Check sheet for the modelled part. Datum: model origin and axes. Units: mm. A direction names the side the tool comes from. Give positions to 0.01 mm unless a question says otherwise; leave off trailing zeros. Write each loop counter-clockwise with the first axis right and the second up, starting at its lowest first coordinate (ties: lowest second). Pieces come first, ordered by that corner, then holes. Notation, with made-up numbers: (-30.75, 60) -> (15.25, 60) arc R26 cw to (15.25, 79) -> close; hole circle Ø11 at (-10.5, 60.5). An arc over 180 degrees is marked (long way). Answer as a JSON object with one key per item and string values.
from build123d import *

# Parameters (mm, degrees)
SKETCH1_W            = 127
SKETCH1_H            = 101.6
BOSS_EXTRUDE1_DEPTH  = 76.2
SKETCH2_R            = 6.35
BOSS_EXTRUDE3_DEPTH  = 50.8
LPATTERN2_COUNT      = 3
LPATTERN2_PITCH      = 15.24
LPATTERN2_COUNT_DIR2 = 3
LPATTERN2_PITCH_DIR2 = 15.24


with BuildPart() as part:
    # Sketch1 → Boss-Extrude1 (new body)
    with BuildSketch(Plane.XY):
        with Locations((63.5, -50.8)):
            Rectangle(SKETCH1_W, SKETCH1_H)
    extrude(amount=BOSS_EXTRUDE1_DEPTH)

    # Sketch2 → Boss-Extrude3 (add)
    with BuildSketch(Plane(origin=(0, 0, 0), x_dir=(1, 0, 0), z_dir=(0, 1, 0))):
        with Locations(Location((68.819241674, -37.547351514, 0), (0, 0, 90))):
            Circle(SKETCH2_R)
    boss_extrude3 = extrude(amount=BOSS_EXTRUDE3_DEPTH)

    # LPattern2: Boss-Extrude3 3 × 3, 1 skipped
    with Locations(*[(-i * LPATTERN2_PITCH, 0, j * LPATTERN2_PITCH_DIR2) for i in range(LPATTERN2_COUNT) for j in range(LPATTERN2_COUNT_DIR2) if (i, j) not in ((0, 0), (1, 1))]):
        add(boss_extrude3)


solid = part.part
1. Access from +Z, -Z, +X, -X, +Y, -Y to the whole of each face (thin tool, end or side, straight path). Record for faces 4 (the face through (53, 50.8, 68)), 5 (the face through (75, 25, 39)).
Determined:
{"face 4": "+Z, -Z, +X, -X, +Y", "face 5": "+Y"}
2. Sectioned sample at D-D, the plane z = 48.5. Enter the section's corners in (x, y).
Determined:
{"outline": "(0, -101.6) -> (127, -101.6) -> (127, 0) -> (73.5, 0) -> (73.5, 50.8) -> (64.14, 50.8) -> (64.14, 0) -> (43.02, 0) -> (43.02, 50.8) -> (33.66, 50.8) -> (33.66, 0) -> (0, 0) -> close"}
3. Scan lines: L1, parallel to X at y = 6, z = 40.5; L2, parallel to Y at x = 22, z = 18. Record each from-to range of solid material in increasing order. Write a range as [from, to].
Determined:
{"L1": "[32.72, 43.96], [47.96, 59.2], [63.2, 74.44]", "L2": "[-101.6, 0]"}
4. Sectioned sample at B-B, the plane z = 70.5. Enter the section's corners in (x, y), plus the area to 3 significant figures.
Determined:
{"outline": "(0, -101.6) -> (127, -101.6) -> (127, 0) -> (74.67, 0) -> (74.67, 50.8) -> (62.97, 50.8) -> (62.97, 0) -> (59.43, 0) -> (59.43, 50.8) -> (47.73, 50.8) -> (47.73, 0) -> (44.19, 0) -> (44.19, 50.8) -> (32.49, 50.8) -> (32.49, 0) -> (0, 0) -> close", "area": "14,700 mm^2"}
5. Go/stop test with flat-tipped pins: P1, Ø12, axis at x = 66, y = 30, coming from the -Z side; P2, Ø1, axis at x = 113, z = 42, coming from the +Y side. Record where each tip stops, or that it passes through.
Determined:
{"P1": "z = 31.2", "P2": "y = 0"}
6. Mould release check, pull along X, two halves, no side actions. Record for faces 1 (the face through (69, 50.8, 53)), 2 (the face through (127, -52, 38)), 3 (the face through (74.453, 25.044, 65.097)): released by +X, released by -X, zero draft, split by the parting line, or undercut.
Determined:
{"face 1": "zero draft", "face 2": "released by +X", "face 3": "undercut"}
7. Sectioned sample at A-A, the plane x = 41. Enter the section's corners in (y, z), plus the area to 3 significant figures.
Determined:
{"outline": "(-101.6, 0) -> (0, 0) -> (0, 31.78) -> (50.8, 31.78) -> (50.8, 43.31) -> (0, 43.31) -> (0, 47.02) -> (50.8, 47.02) -> (50.8, 58.55) -> (0, 58.55) -> (0, 62.26) -> (50.8, 62.26) -> (50.8, 73.79) -> (0, 73.79) -> (0, 76.2) -> (-101.6, 76.2) -> close", "area": "9,500 mm^2"}
8. Sectioned sample at C-C, the plane x = 77. Enter the section's corners in (y, z).
Determined:
{"outline": "(-101.6, 0) -> (0, 0) -> (0, 76.2) -> (-101.6, 76.2) -> close"}
